The model under review builds one solid part; all positions refer to its coordinate system, in mm. Face numbers are marked on the shaded views. A direction names the side the tool comes from. Round coordinates to 2 decimals unless told otherwise and drop trailing zeros. Loops run counter-clockwise (first coordinate to the right, second up) from the corner with the lowest first, then second, coordinate; pieces in that order, holes last. Notation, with made-up numbers: M 38.25,20.5 L 55.25,20.5 A16 cw 55.25,35.5 Z; hole C 86.25,-0.5 d10. An arc over 180 degrees is marked long. Answer as a JSON object with one key per item and string values. Group by question number.
Item 1: Consider section C-C (y = 4). Give the boundary of the cut face in (x, z), and give its area (3 significant figures).
Item 2: Consider section B-B (z = 0). Give the boundary of the cut face in (x, y).
Item 3: Tool access review of the marked faces 1 and 2: name each direction out of +Z, -Z, +X, -X, +Y, -Y from which nothing blocks a thin tool from reaching the whole face with its end or side.
Item 4: Consider section A-A (x = 0). Give the boundary of the cut face in (y, z), and give its area (3 significant figures).
Item 5: Insertion check: P1, Ø8, axis at x = 0, z = 0, coming from the +Y side; P2, Ø6, axis at x = 5, y = 8.5, coming from the -Z side; P3, Ø10, axis at x = -0.5, z = -7.5, coming from the -Y side; P4, Ø1.5, axis at y = 2.5, z = -5.5, coming from the +X side. Each pin has a flat end and moves straight along its axis. Give the tip position at first contact, or say it passes through.
Item 6: To check wall thickness, follow line 1 (Z direction, x = 0, y = 12); line 2 (X direction, y = 2.25, z = 0); line 3 (X direction, y = 12.75, z = 0). State the ranges of each line that lie inside material, in increasing order.
Item 7: The part is to be moulded in two halves that separate along X. For the marked faces 3, 4 and 5, say which applies: +X half, -X half, draft (parallel to the pull), parting line (faces both ways), or undercut.
Item 8: Consider section D-D (z = 6.5). Give the boundary of the cut face in (x, y).
```python
from build123d import *

# Parameters (mm, degrees)
SKETCH1_R           = 14.69
BOSS_EXTRUDE1_DEPTH = 14
SKETCH2_R           = 11.1
CUT_EXTRUDE1_DEPTH  = 7.4
SKETCH3_R           = 16.09
SKETCH3_R_2         = 14.69
BOSS_EXTRUDE2_DEPTH = 1.4
SKETCH4_R           = 3.5
CUT_EXTRUDE2_DEPTH  = 7.6


with BuildPart() as part:
    # Sketch1 → Boss-Extrude1 (new body)
    with BuildSketch(Plane(origin=(0, 0, 0), x_dir=(1, 0, 0), z_dir=(0, 1, 0))):
        Circle(SKETCH1_R)
    extrude(amount=BOSS_EXTRUDE1_DEPTH)

    # Sketch2 → Cut-Extrude1 (cut)
    with BuildSketch(Plane(origin=(0, 14, 0), x_dir=(1, 0, 0), z_dir=(0, 1, 0))):
        Circle(SKETCH2_R)
    extrude(amount=-CUT_EXTRUDE1_DEPTH, mode=Mode.SUBTRACT)

    # Sketch3 → Boss-Extrude2 (add)
    with BuildSketch(Plane(origin=(0, 14, 0), x_dir=(1, 0, 0), z_dir=(0, 1, 0))):
        Circle(SKETCH3_R)
        Circle(SKETCH3_R_2, mode=Mode.SUBTRACT)
    extrude(amount=-BOSS_EXTRUDE2_DEPTH)

    # Sketch4 → Cut-Extrude2 (cut, through all)
    with BuildSketch(Plane(origin=(0, 6.6, 0), x_dir=(1, 0, 0), z_dir=(0, 1, 0))):
        Circle(SKETCH4_R)
    extrude(amount=-CUT_EXTRUDE2_DEPTH, mode=Mode.SUBTRACT)


solid = part.part
```
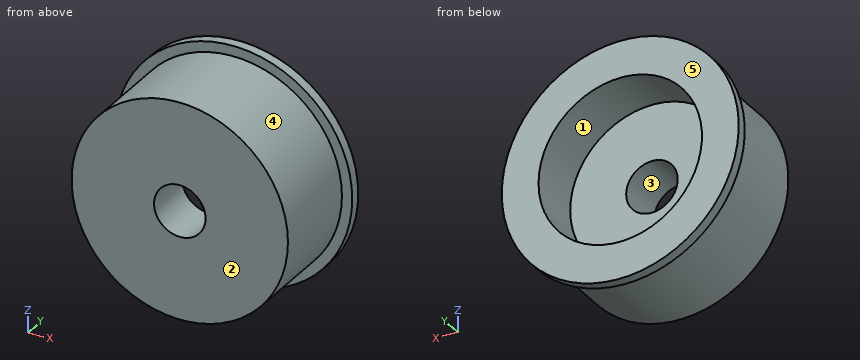
Geometry results:
{
 "1": {"outline": "C 0,0 d29.38; hole C 0,0 d7", "area": "639 mm^2"},
 "2": {"outline": "M -16.09,12.6 L -14.69,12.6 L -14.69,0 L -3.5,0 L -3.5,6.6 L -11.1,6.6 L -11.1,14 L -16.09,14 Z; M 3.5,0 L 14.69,0 L 14.69,12.6 L 16.09,12.6 L 16.09,14 L 11.1,14 L 11.1,6.6 L 3.5,6.6 Z"},
 "3": {"face 1": "+Y", "face 2": "+Z, -Z, +X, -X, -Y"},
 "4": {"outline": "M 0,-14.69 L 12.6,-14.69 L 12.6,-16.09 L 14,-16.09 L 14,-11.1 L 6.6,-11.1 L 6.6,-3.5 L 0,-3.5 Z; M 0,3.5 L 6.6,3.5 L 6.6,11.1 L 14,11.1 L 14,16.09 L 12.6,16.09 L 12.6,14.69 L 0,14.69 Z", "area": "205 mm^2"},
 "5": {"P1": "stops at y = 6.6", "P2": "stops at z = -14.55", "P3": "stops at y = 0", "P4": "stops at x = 13.9"},
 "6": {"line 1": "z = -14.69 to -11.1, 11.1 to 14.69", "line 2": "x = -14.69 to -3.5, 3.5 to 14.69", "line 3": "x = -16.09 to -11.1, 11.1 to 16.09"},
 "7": {"face 3": "undercut", "face 4": "parting line", "face 5": "draft"},
 "8": {"outline": "M -14.72,12.6 L -13.17,12.6 L -13.17,0 L 13.17,0 L 13.17,12.6 L 14.72,12.6 L 14.72,14 L 9,14 L 9,6.6 L -9,6.6 L -9,14 L -14.72,14 Z"}
}
